Job drawing, mm, ordinate dimensions from the low corner. One solid piece. A direction names the side the tool comes from. Give positions to 0.01 mm unless a question says otherwise; leave off trailing zeros. Loops run counter-clockwise (first coordinate to the right, second up) from the corner with the lowest first, then second, coordinate; pieces in that order, holes last. Notation, with made-up numbers: M -1.75,5.5 L 45.25,5.5 A21 cw 45.25,22.5 Z; hole C 6.25,-5.5 d9. An arc over 180 degrees is marked long. Answer in a Markdown table with one row per item.
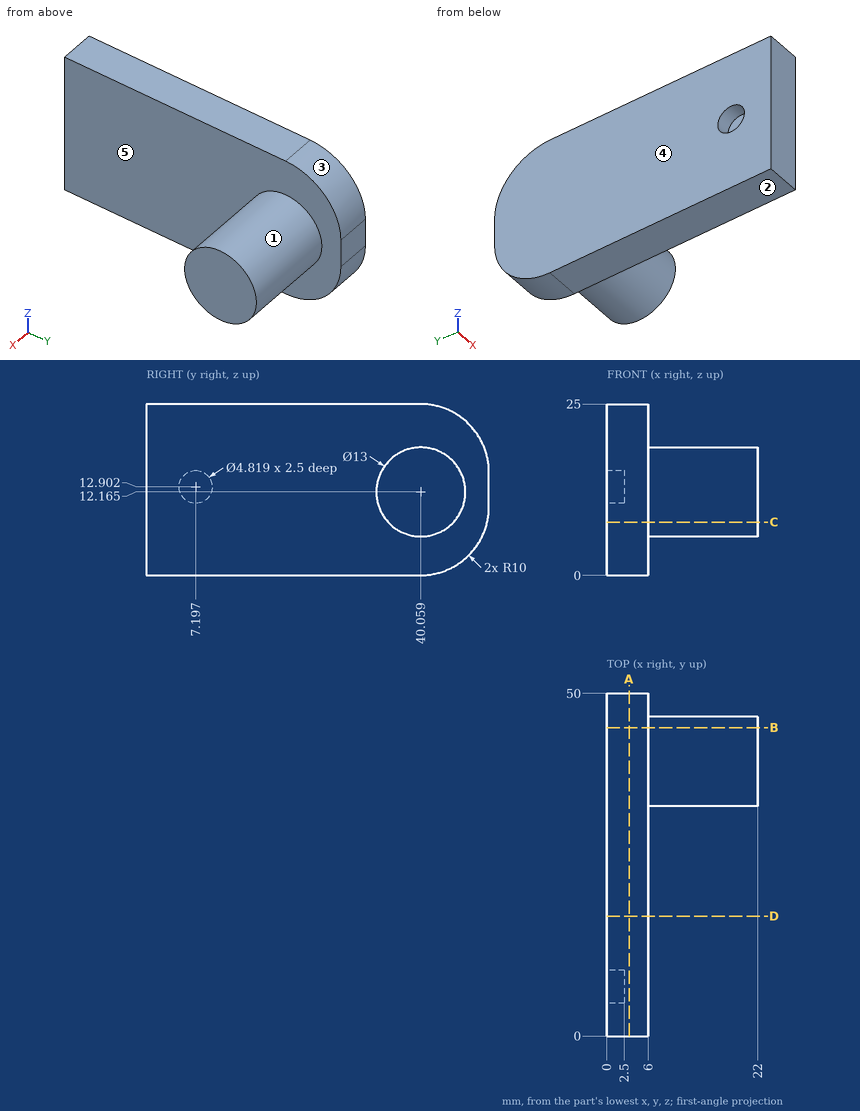
(1) Drill centre lines: line 1 along X through (y, z) = (7, 13); line 2 along X through (y, z) = (17, 12); line 3 along Y through (x, z) = (5, 20.5). Where is each one in solid material? Low to high.
Recorded:
| item | result |
|---|---|
| line 1 | x = 2.5 to 6 |
| line 2 | x = 0 to 6 |
| line 3 | y = 0 to 48.35 |
(2) Pull direction X, two halves, no side cores. Call the marked faces 3, 4 and 5: +X half, -X half, draft (parallel to the pull), parting line (faces both ways), or undercut.
Recorded:
| item | result |
|---|---|
| face 3 | draft |
| face 4 | -X half |
| face 5 | +X half |
(3) Which spindle directions (+Z, -Z, +X, -X, +Y, -Y) get a long thin tool onto all of the face, cutting with end or side? Do the marked faces 1 and 2. Say none if no direction does.
Recorded:
| item | result |
|---|---|
| face 1 | +X |
| face 2 | -Z, +X, -X, +Y, -Y |
(4) Saw through at A-A (x = 3.25). Write the cut outline in (y, z), plus the area to 3 significant figures.
Recorded:
| item | result |
|---|---|
| outline | M 0,0 L 40,0 A10 ccw 50,10 L 50,15 A10 ccw 40,25 L 0,25 Z |
| area | 1,210 mm^2 |
(5) Saw through at C-C (z = 7.75). Write the cut outline in (x, y), plus the area to 3 significant figures.
Recorded:
| item | result |
|---|---|
| outline | M 0,0 L 6,0 L 6,35.29 L 22,35.29 L 22,44.83 L 6,44.83 L 6,49.74 L 0,49.74 Z |
| area | 451 mm^2 |
(6) Pin check, flat tips, straight feed: pin 1 Ø1 at (y, z) = (10.5, 18) entering from +X; pin 2 Ø12 at (x, z) = (17, 14.5) entering from -Y; pin 3 Ø4 at (y, z) = (34, 16) entering from -X; pin 4 Ø1.5 at (x, z) = (10.5, 7.5) entering from +Y. Stop position of each tip, or through.
Recorded:
| item | result |
|---|---|
| pin 1 | stops at x = 6 |
| pin 2 | stops at y = 33.56 |
| pin 3 | stops at x = 0 |
| pin 4 | stops at y = 45.25 |
(7) Saw through at B-B (y = 45). Write the cut outline in (x, z).
Recorded:
| item | result |
|---|---|
| outline | M 0,1.34 L 6,1.34 L 6,7.94 L 22,7.94 L 22,16.39 L 6,16.39 L 6,23.66 L 0,23.66 Z |
(8) Saw through at D-D (y = 17.5). Write the cut outline in (x, z).
Recorded:
| item | result |
|---|---|
| outline | M 0,0 L 6,0 L 6,25 L 0,25 Z |
